The figure shows three views and two pictorial views of one solid part (mm, origin at its lowest corner). Answer the questions. Coordinates: 2 decimals unless noted, no trailing zeros. Write each loop counter-clockwise with the first axis right and the second up, starting at its lowest first coordinate (ties: lowest second). Pieces come first, ordered by that corner, then holes. Notation, with made-up numbers: M -39,58.25 L -16,58.25 A15 ccw -16,76.25 Z; hole C 20,1.5 d6. An arc over 180 degrees is marked long. Use a Markdown table: item, result. Add a question column.
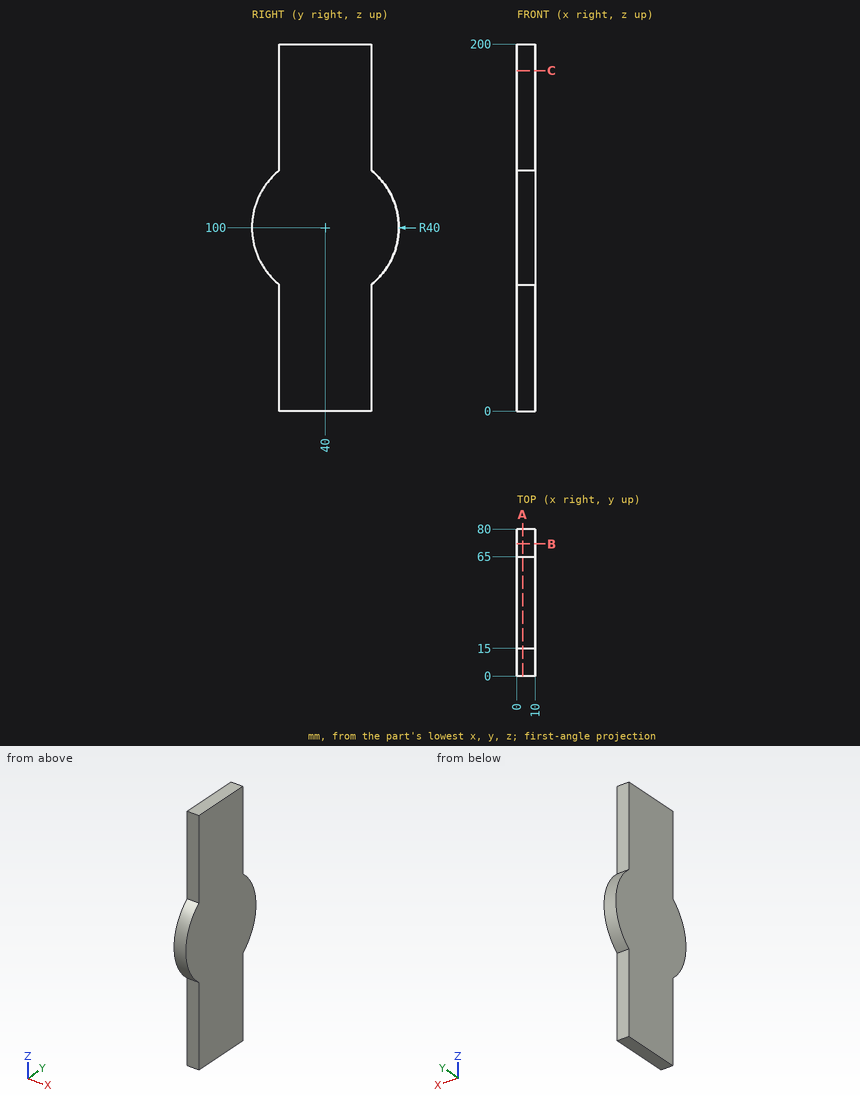
Item 1: Find section A-A on x = 3.25. Give the vertices of the cut face in (y, z), then the cut area to 3 significant figures.
Item 2: Each of these flat-tipped pins is pushed along its axis until it touches: pin 1 (2 mm diameter, centred on x = 8.5, z = 81.5, fed in from -Y); pin 2 (3 mm diameter, centred on x = 4, z = 41.5, fed in from -Y); pin 3 (2 mm diameter, centred on x = 4, z = 118.5, fed in from +Y). Where does it stop, or does it pass through?
Item 3: Consider probe 1 along Y at (x, z) = (7.75, 141); probe 2 along Y at (x, z) = (3.75, 131); probe 3 along Z at (x, y) = (8.75, 8). Determine where each line is inside the solid, lowest interval first.
Item 4: Find section C-C on z = 185.5. Give the vertices of the cut face in (x, y).
Item 5: Find section B-B on y = 72. Give the vertices of the cut face in (x, z), then the cut area to 3 significant figures.
Geometry says:
| question | item | result |
|---|---|---|
| 1 | outline | M 15,0 L 65,0 L 65,68.78 A40 ccw 65,131.22 L 65,200 L 15,200 L 15,131.22 A40 ccw 15,68.78 Z |
| 1 | area | 11,300 mm2 |
| 2 | pin 1 | stops at y = 4.03 |
| 2 | pin 2 | stops at y = 15 |
| 2 | pin 3 | stops at y = 75.97 |
| 3 | probe 1 | y = 15 to 65 |
| 3 | probe 2 | y = 14.72 to 65.28 |
| 3 | probe 3 | z = 76 to 124 |
| 4 | outline | M 0,15 L 10,15 L 10,65 L 0,65 Z |
| 5 | outline | M 0,76 L 10,76 L 10,124 L 0,124 Z |
| 5 | area | 480 mm2 |
